```python
from build123d import *

# Parameters (mm, degrees)
F0_W      = 50.710565
F0_H      = 50.99229
F1_DEPTH  = 25.4
F1_FACE_W = 50.710564
F1_FACE_H = 50.99229
F2_DEPTH  = 76.2
F4_DEPTH  = 76.2


with BuildPart() as f1:
    # F0 (on Right) → F1 (new body)
    with BuildSketch(Plane.YZ):
        with Locations((10.5647, 5.352781)):
            Rectangle(F0_W, F0_H)
    extrude(amount=F1_DEPTH)

    # F1_face (on face) → F2 (join)
    with BuildSketch(Plane(origin=(25.4, 10.564701, 5.352781), x_dir=(0, 1, 0), z_dir=(1, 0, 0))):
        Rectangle(F1_FACE_W, F1_FACE_H)
    extrude(amount=-F2_DEPTH)

    # F3 (on face) → F4 (cut)
    with BuildSketch(Plane(origin=(0, 0, -20.143364), x_dir=(1, 0, 0), z_dir=(0, 0, -1))):
        with BuildLine():
            ThreePointArc((3.819773, -10.564701), (-1.018756, 1.116543), (-12.7, 5.955072))
            Line((-12.7, 5.955072), (-12.7, -10.564701))
            Line((-12.7, -10.564701), (3.819773, -10.564701))
        make_face()
        with BuildLine():
            Line((-12.7, -10.564701), (-12.7, 5.955072))
            ThreePointArc((-12.7, 5.955072), (-24.381244, 1.116543), (-29.219773, -10.564701))
            Line((-29.219773, -10.564701), (-12.7, -10.564701))
        make_face()
        with BuildLine():
            Line((3.819773, -10.564701), (-12.7, -10.564701))
            Line((-12.7, -10.564701), (-12.7, -27.084474))
            ThreePointArc((-12.7, -27.084474), (-1.018756, -22.245944), (3.819773, -10.564701))
        make_face()
        with BuildLine():
            Line((-12.7, -27.084474), (-12.7, -10.564701))
            Line((-12.7, -10.564701), (-29.219773, -10.564701))
            ThreePointArc((-29.219773, -10.564701), (-24.381244, -22.245944), (-12.7, -27.084474))
        make_face()
    extrude(amount=-F4_DEPTH, mode=Mode.SUBTRACT)


solid = f1.part
```
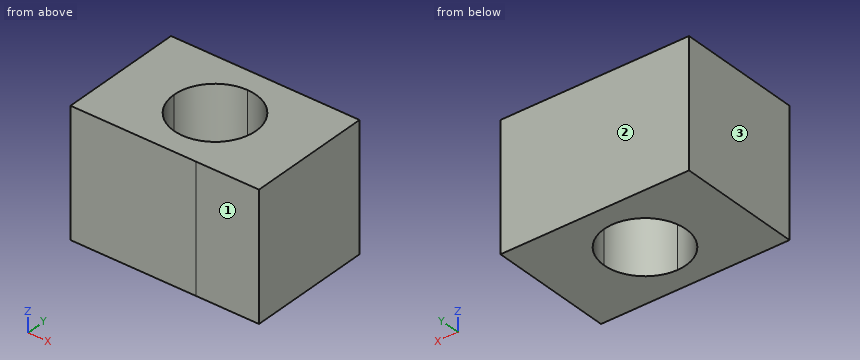
Model file for the job. Use its own axes, mm. Face numbers are marked on the shaded views. Round coordinates to 2 decimals unless told otherwise and drop trailing zeros. Write each loop counter-clockwise with the first axis right and the second up, starting at its lowest first coordinate (ties: lowest second). Pieces come first, ordered by that corner, then holes. Notation, with made-up numbers: M 37,-30.5 L 44,-30.5 A6 ccw 44,-26.5 Z; hole C -32.5,-28 d6. An arc over 180 degrees is marked long. Put each result on its own line as item: value.
Item 1: Cut at B-B (y = 4). List the corners of the cut face in (x, z).
Responses:
outline: M -50.8,-20.14 L -27.86,-20.14 L -27.86,30.85 L -50.8,30.85 Z; M 2.46,-20.14 L 25.4,-20.14 L 25.4,30.85 L 2.46,30.85 Z
Item 2: Mould opens along Y. For the marked faces 1, 2 and 3 say: +Y half, -Y half, draft (parallel to the pull), parting line (faces both ways), or undercut.
Responses:
face 1: -Y half
face 2: +Y half
face 3: draft
Item 3: Probe L1, parallel to X at y = 6.5, z = 27; L2, parallel to X at y = 13.5, z = 23.5; L3, parallel to Y at x = -26.5, z = -3. List the from-to ranges inside material, lowest first. Write a range as from..to.
Responses:
L1: -50.8..-28.71, 3.31..25.4
L2: -50.8..-28.96, 3.56..25.4
L3: -14.79..1.48, 19.65..35.92
Item 4: Cut at C-C (x = -4). List the corners of the cut face in (y, z), and give its area (3 significant figures).
Responses:
outline: M -14.79,-20.14 L -3.48,-20.14 L -3.48,30.85 L -14.79,30.85 Z; M 24.61,-20.14 L 35.92,-20.14 L 35.92,30.85 L 24.61,30.85 Z
area: 1,150 mm²
